```python
from build123d import *

# Parameters (mm, degrees)
F0_W     = 13.97
F0_H     = 6.35
F1_DEPTH = 12.7
F2_R     = 6.35
F3_DEPTH = 25.4


with BuildPart() as f1:
    # F0 (on Front) → F1 (new body)
    with BuildSketch(Plane.XZ):
        Polygon((-13.97, 27.432009), (-13.97, 33.782009), (-13.97, 45.466005), (-64.77, 45.466005), (-64.77, 34.602262), (-64.77, 25.704423), (-64.77, 13.716005), (-13.97, 13.716005), align=None)
        Polygon((0, 45.466005), (0, 33.782009), (0, 27.432009), (0, 13.716005), (50.8, 13.716005), (50.8, 29.591005), (50.8, 35.010789), (50.8, 45.466005), align=None)
        with Locations((-6.985, 30.607009)):
            Rectangle(F0_W, F0_H)
    extrude(amount=F1_DEPTH)

    # F2 (on face) → F3 (cut)
    with BuildSketch(Plane.XZ.offset(12.7)):
        with Locations((-41.964256, 29.434583)):
            Circle(F2_R)
        with Locations((24.473708, 29.912554)):
            Circle(F2_R)
    extrude(amount=-F3_DEPTH, mode=Mode.SUBTRACT)


solid = f1.part
```
Read the model definition and answer for the solid it produces. Units are mm, in the model's axes. A direction names the side the tool comes from. Round coordinates to 2 decimals unless told otherwise and drop trailing zeros. Write each loop counter-clockwise with the first axis right and the second up, starting at its lowest first coordinate (ties: lowest second). Pieces come first, ordered by that corner, then holes. Notation, with made-up numbers: (15, -26) - (26, -26) arc R14 ccw to (26, -14) - close; hole circle Ø4 at (31.5, 81.25). An arc over 180 degrees is marked (long way). One line per item, written item: value.
Q1. Straight lines are drawn through the part: line 1 (X direction, y = -5.5, z = 29.5); line 2 (X direction, y = -1.25, z = 17); line 3 (X direction, y = -4.5, z = 31). For each, find the intervals that lie inside material, in ascending order. Write a range as from..to.
The answers:
line 1: x = -64.77..-48.31, -35.61..18.14, 30.81..50.8
line 2: x = -64.77..-13.97, 0..50.8
line 3: x = -64.77..-48.12, -35.81..18.22, 30.73..50.8
Q2. Which of the six approach directions +Z, -Z, +X, -X, +Y, -Y give full straight-line access (tool end or side, diameter ignored) to faces 4 (the flat face through (-13.97, -6, 20)), 5 (the flat face through (-40, -6, 13.716)), 6 (the flat face through (-7, -6, 33.782))?
The answers:
face 4: -Z, +Y, -Y
face 5: -Z, +X, -X, +Y, -Y
face 6: +Z, +Y, -Y
Q3. Find section D-D (z = 26). Determine the outline of the cut face in (x, y).
The answers:
outline: (-64.77, -12.7) - (-47.31, -12.7) - (-47.31, 0) - (-64.77, 0) - close; (-36.62, -12.7) - (-13.97, -12.7) - (-13.97, 0) - (-36.62, 0) - close; (0, -12.7) - (19.47, -12.7) - (19.47, 0) - (0, 0) - close; (29.48, -12.7) - (50.8, -12.7) - (50.8, 0) - (29.48, 0) - close
Q4. Find section C-C (y = -2.5). Determine the outline of the cut face in (x, z).
The answers:
outline: (-64.77, 13.72) - (-13.97, 13.72) - (-13.97, 27.43) - (0, 27.43) - (0, 13.72) - (50.8, 13.72) - (50.8, 45.47) - (0, 45.47) - (0, 33.78) - (-13.97, 33.78) - (-13.97, 45.47) - (-64.77, 45.47) - close; hole circle Ø12.7 at (-41.96, 29.43); hole circle Ø12.7 at (24.47, 29.91)
Q5. Find section B-B (x = -42). Determine the outline of the cut face in (y, z).
The answers:
outline: (-12.7, 13.72) - (0, 13.72) - (0, 23.08) - (-12.7, 23.08) - close; (-12.7, 35.78) - (0, 35.78) - (0, 45.47) - (-12.7, 45.47) - close
Q6. For a pull along Z with two mould halves and no side action, classify faces 1 (the flat face through (-13.97, -6, 40)), 2 (the flat face through (-7, -6, 27.432)), 3 (the cylindrical face through (-42.79, -6.44, 35.73)) as pulls with the +Z half, pulls with the -Z half, needs draft (parallel to the pull), parting line crosses it, or undercut.
The answers:
face 1: needs draft
face 2: pulls with the -Z half
face 3: undercut
Q7. Each of these flat-tipped pins is pushed along its axis until it touches: P1, Ø4, axis at x = -5.5, y = -6, coming from the -Z side; P2, Ø6.5, axis at x = -4.5, y = -9, coming from the +Z side. Where does it stop, or does it pass through?
The answers:
P1: stops at z = 27.43
P2: stops at z = 33.78
Q8. Find section A-A (z = 41). Determine the outline of the cut face in (x, y).
The answers:
outline: (-64.77, -12.7) - (-13.97, -12.7) - (-13.97, 0) - (-64.77, 0) - close; (0, -12.7) - (50.8, -12.7) - (50.8, 0) - (0, 0) - close
